Build history of the part. All positions in model axes, mm. Give positions to 0.01 mm unless a question says otherwise; leave off trailing zeros. Loops run counter-clockwise (first coordinate to the right, second up) from the corner with the lowest first, then second, coordinate; pieces in that order, holes last. Notation, with made-up numbers: (87, -6) -> (141, -6) arc R30 ccw to (141, 17) -> close; hole circle Ø11 at (25, 28.5). An arc over 180 degrees is marked (long way). Answer as a JSON object with one key per item and string values. Group by question number.
Q1. Band-saw the part on C-C, the plane z = -149.5. Write the cut outline in (x, y), plus the area to 3 significant figures.
Q2. Band-saw the part on A-A, the plane z = -194. Write the cut outline in (x, y).
Q3. Drop flat-ended pins along their axis: pin 1 (1.9 mm diameter, centred on x = 2, y = -320, fed in from +Z); pin 2 (6 mm diameter, centred on y = -38.1, z = -9.525, fed in from +X). Give the stop position or say it passes through.
Q4. Band-saw the part on B-B, the plane x = 2.5. Count the separate pieces of the cut face and the enclosed holes in it, plus the area to 3 significant figures.
Q5. Wall check: probe 1 along Y at (x, z) = (5, -28.5); probe 2 along Z at (x, y) = (3.5, -86); probe 3 along Z at (x, y) = (4.5, -406.4). Give the ranges that are in metal, low to high. Write a range as from..to.
from build123d import *

# Parameters (mm, degrees)
BOSS_EXTRUDE1_DEPTH     = 6.35
SKETCH2_R               = 3.3655
CUT_EXTRUDE1_DEPTH      = 7.35
FILLET1_R               = 6.35
CUT_EXTRUDE6_DEPTH      = 7.35
SKETCH4_R               = 3.3655
CUT_EXTRUDE3_DEPTH      = 7.35
CUT_EXTRUDE7_DEPTH      = 7.35
CUT_EXTRUDE8_DEPTH      = 1
CUT_EXTRUDE8_DEPTH_BACK = 7.35
SKETCH8_W               = 50.8
SKETCH8_H               = 50.8
CUT_EXTRUDE9_DEPTH      = 7.35
FILLET2_R               = 6.35


with BuildPart() as part:
    # Sketch1 → Boss-Extrude1 (new body)
    with BuildSketch(Plane(origin=(0, 0, 0), x_dir=(0, 0, -1), z_dir=(1, 0, 0))):
        with BuildLine():
            Line((0, 0), (0, -609.6))
            Line((0, -609.6), (76.2, -609.6))
            ThreePointArc((76.2, -609.6), (219.884097937, -550.084097937), (279.4, -406.4))
            Line((279.4, -406.4), (279.4, 0))
            Line((279.4, 0), (0, 0))
        make_face()
    extrude(amount=BOSS_EXTRUDE1_DEPTH)

    # Sketch2 → Cut-Extrude1 (cut, through all)
    with BuildSketch(Plane(origin=(6.35, 0, 0), x_dir=(0, 0, -1), z_dir=(1, 0, 0))):
        with Locations((266.7, -17.78)):
            Circle(SKETCH2_R)
        with Locations((12.7, -596.9)):
            Circle(SKETCH2_R)
        with Locations((210.903841816, -541.103841816)):
            Circle(SKETCH2_R)
        with Locations((19.05, -17.78)):
            Circle(SKETCH2_R)
    extrude(amount=-CUT_EXTRUDE1_DEPTH, mode=Mode.SUBTRACT)

    # Fillet1
    fillet1_edges = [part.edges().sort_by_distance(p)[0] for p in [
        (3.175, 0, -279.4),
        (3.175, -609.6, 0),
        (3.175, 0, 0),
    ]]
    fillet(fillet1_edges, radius=FILLET1_R)

    # Sketch3 → Cut-Extrude6 (cut, through all)
    with BuildSketch(Plane(origin=(6.35, 0, 0), x_dir=(0, 0, -1), z_dir=(1, 0, 0))):
        with BuildLine():
            Line((63.5, -7.62), (114.3, -7.62))
            ThreePointArc((114.3, -7.62), (116.205, -9.525), (114.3, -11.43))
            Line((114.3, -11.43), (63.5, -11.43))
            ThreePointArc((63.5, -11.43), (61.595, -9.525), (63.5, -7.62))
        make_face()
        with BuildLine():
            Line((165.1, -7.62), (215.9, -7.62))
            ThreePointArc((215.9, -7.62), (217.805, -9.525), (215.9, -11.43))
            Line((215.9, -11.43), (165.1, -11.43))
            ThreePointArc((165.1, -11.43), (163.195, -9.525), (165.1, -7.62))
        make_face()
    extrude(amount=-CUT_EXTRUDE6_DEPTH, mode=Mode.SUBTRACT)

    # Sketch4 → Cut-Extrude3 (cut, through all)
    with BuildSketch(Plane(origin=(6.35, 0, 0), x_dir=(0, 0, -1), z_dir=(1, 0, 0))):
        with Locations((9.525, -38.1)):
            Circle(SKETCH4_R)
        with Locations((9.525, -406.4)):
            Circle(SKETCH4_R)
        with Locations((9.525, -571.5)):
            Circle(SKETCH4_R)
    extrude(amount=-CUT_EXTRUDE3_DEPTH, mode=Mode.SUBTRACT)

    # Sketch6 → Cut-Extrude7 (cut, through all)
    with BuildSketch(Plane(origin=(6.35, 0, 0), x_dir=(0, 0, -1), z_dir=(1, 0, 0))):
        with BuildLine():
            Line((260.35, -65.0875), (260.35, -169.8625))
            ThreePointArc((260.35, -169.8625), (258.445, -171.7675), (256.54, -169.8625))
            Line((256.54, -169.8625), (256.54, -65.0875))
            ThreePointArc((256.54, -65.0875), (258.445, -63.1825), (260.35, -65.0875))
        make_face()
        with BuildLine():
            Line((256.54, -379.4125), (256.54, -274.6375))
            ThreePointArc((256.54, -274.6375), (258.445, -272.7325), (260.35, -274.6375))
            Line((260.35, -274.6375), (260.35, -379.4125))
            ThreePointArc((260.35, -379.4125), (258.445, -381.3175), (256.54, -379.4125))
        make_face()
    extrude(amount=-CUT_EXTRUDE7_DEPTH, mode=Mode.SUBTRACT)

    # Sketch7 → Cut-Extrude8 (cut, two sides)
    with BuildSketch(Plane(origin=(6.35, 0, 0), x_dir=(0, 0, -1), z_dir=(1, 0, 0))) as cut_extrude8_sk:
        with BuildLine():
            Line((9.525, -586.74), (41.275, -586.74))
            ThreePointArc((41.275, -586.74), (43.18, -588.645), (41.275, -590.55))
            Line((41.275, -590.55), (9.525, -590.55))
            ThreePointArc((9.525, -590.55), (7.62, -588.645), (9.525, -586.74))
        make_face()
    extrude(amount=CUT_EXTRUDE8_DEPTH, mode=Mode.SUBTRACT)
    extrude(cut_extrude8_sk.sketch, amount=-CUT_EXTRUDE8_DEPTH_BACK, mode=Mode.SUBTRACT)

    # Sketch8 → Cut-Extrude9 (cut, through all)
    with BuildSketch(Plane(origin=(6.35, 0, 0), x_dir=(0, 0, -1), z_dir=(1, 0, 0))):
        with Locations((25.4, -292.1)):
            Rectangle(SKETCH8_W, SKETCH8_H)
    extrude(amount=-CUT_EXTRUDE9_DEPTH, mode=Mode.SUBTRACT)

    # Fillet2
    fillet2_edges = [part.edges().sort_by_distance(p)[0] for p in [
        (3.175, -317.5, 0),
        (3.175, -266.7, 0),
        (3.175, -266.7, -50.8),
        (3.175, -317.5, -50.8),
    ]]
    fillet(fillet2_edges, radius=FILLET2_R)


solid = part.part
Worked answers:
{
 "1": {"outline": "(0, -595.92) -> (6.35, -595.92) -> (6.35, 0) -> (0, 0) -> close", "area": "3,780 mm2"},
 "2": {"outline": "(0, -571.97) -> (6.35, -571.97) -> (6.35, -11.43) -> (0, -11.43) -> close; (0, -7.62) -> (6.35, -7.62) -> (6.35, 0) -> (0, 0) -> close"},
 "3": {"pin 1": "z = -0.7", "pin 2": "through"},
 "4": {"separate pieces": "1", "enclosed holes": "12", "area": "157,000 mm2"},
 "5": {"probe 1": "-609.6..-590.55, -586.74..-317.5, -266.7..0", "probe 2": "-279.4..-260.35, -256.54..0", "probe 3": "-279.4..-12.89, -6.16..0"}
}
